For this review, use the dimensioned drawing (mm, ordinates from the lowest corner) and the shaded views. A direction names the side the tool comes from. Coordinates: 2 decimals unless noted, no trailing zeros. Write each loop counter-clockwise with the first axis right and the second up, starting at its lowest first coordinate (ties: lowest second). Pieces come first, ordered by that corner, then holes. Notation, with made-up numbers: M 14,69 L 33,69 A29 ccw 33,102 Z; hole C 44.25,59 d11. An arc over 180 degrees is marked long. One line per question, with ' | ' between items.
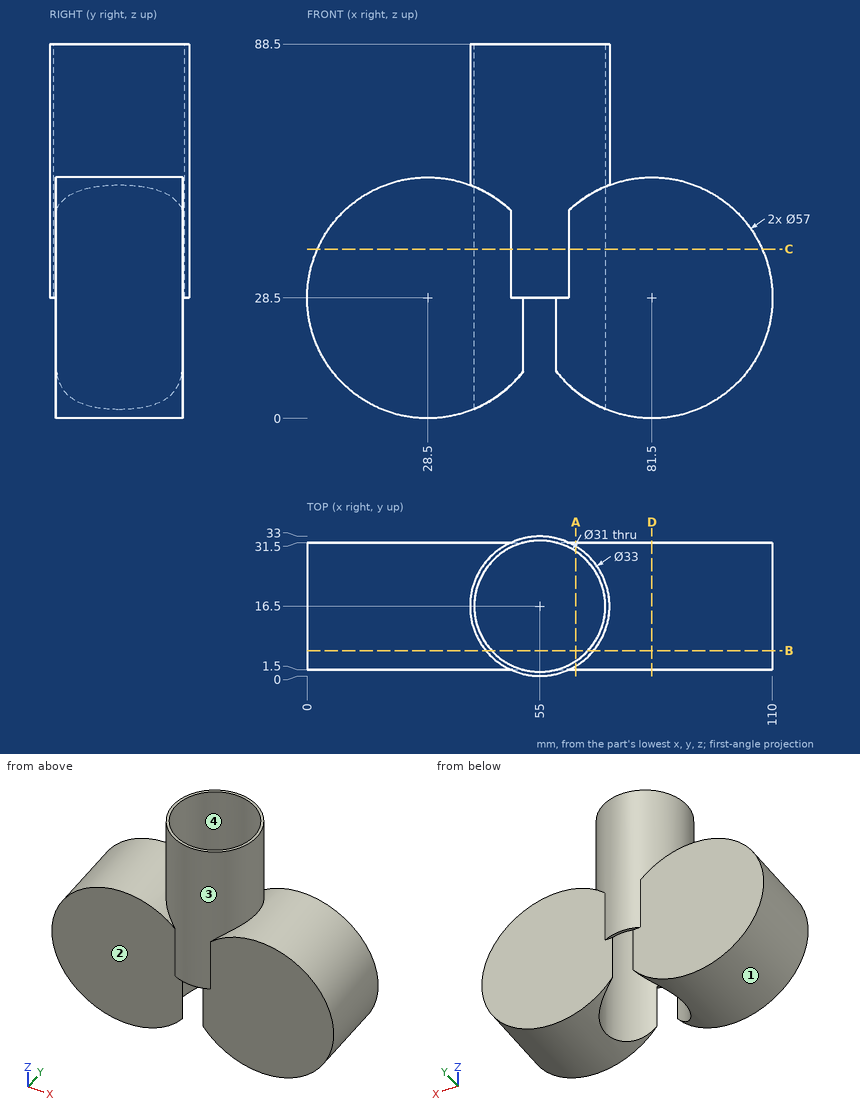
1) We need section C-C on z = 40. State the section outline as (x, y) points, then the cut area to 3 significant figures.
Responses:
outline: M 2.42,1.5 L 48.13,1.5 A16.5 ccw 61.87,1.5 L 107.58,1.5 L 107.58,31.5 L 61.87,31.5 A16.5 ccw 48.13,31.5 L 2.42,31.5 Z; hole C 55,16.5 d31 | area: 2,430 mm^2
2) We need section B-B on y = 6. State the section outline as (x, z) points.
Responses:
outline: M 42.27,53.45 A28.5 ccw long 43.6,4.33 L 43.6,88.5 L 42.27,88.5 Z; M 66.4,4.33 A28.5 ccw long 67.73,53.45 L 67.73,88.5 L 66.4,88.5 Z
3) The part is to be moulded in two halves that separate along X. For the marked faces 1 and 2, say which applies: +X half, -X half, draft (parallel to the pull), parting line (faces both ways), or undercut.
Responses:
face 1: undercut | face 2: draft
4) We need section D-D on x = 81.5. State the section outline as (y, z) points.
Responses:
outline: M 1.5,0 L 31.5,0 L 31.5,57 L 1.5,57 Z
5) To check wall thickness, follow line 1 along Y through (x, z) = (55, 61); line 2 along Y through (x, z) = (87, 54); line 3 along X through (y, z) = (21, 23.5). State the ranges of each line that lie inside material, in increasing order. Write a range as [from, to].
Responses:
line 1: [0, 1], [32, 33] | line 2: [1.5, 31.5] | line 3: [0.44, 40.17], [69.83, 109.56]
6) Machinability: for the marked faces 3 and 4, which of the approach directions +Z, -Z, +X, -X, +Y, -Y give a long, thin tool a straight path to every point of the face, cutting with its end or side? Answer none if there is none.
Responses:
face 3: +Z | face 4: +Z, -Z
7) Insertion check: pin 1 Ø3 at (x, z) = (73.5, 19.5) entering from +Y; pin 2 Ø1.5 at (x, y) = (87, 25.5) entering from +Z; pin 3 Ø10 at (x, y) = (53.5, 7) entering from +Z; pin 4 Ø3 at (x, y) = (28.5, 18) entering from -Z. Each pin has a flat end and moves straight along its axis. Give the tip position at first contact, or say it passes through.
Responses:
pin 1: y = 31.5 | pin 2: z = 56.6 | pin 3: through | pin 4: z = 0
8) We need section A-A on x = 63.5. State the section outline as (y, z) points, then the cut area to 3 significant figures.
Responses:
outline: M 1.5,6.4 L 3.54,6.4 L 3.54,88.5 L 2.36,88.5 L 2.36,50.6 L 1.5,50.6 Z; M 29.46,6.4 L 31.5,6.4 L 31.5,50.6 L 30.64,50.6 L 30.64,88.5 L 29.46,88.5 Z | area: 270 mm^2
